Autodesk Inventor part; units mm, degrees
ref_plane "YZ Plane" through (0, 0, 0) normal (1, 0, 0) x (0, 1, 0)
ref_plane "XZ Plane" through (0, 0, 0) normal (0, 1, 0) x (-1, 0, 0)
ref_plane "XY Plane" through (0, 0, 0) normal (0, 0, 1) x (1, 0, 0)
sketch "Szkic1" plane through (0, 0, 0) normal (1, 0, 0) x (0, 1, 0)
  circle A0 centre (0, 0) radius 8
  dimension "d0" = 16
extrude "Wyciągnięcie proste1" add sketch "Szkic1" along normal mid plane 15
sketch "Szkic2" plane through (7.5, 0, 0) normal (1, 0, 0) x (0, 0, -1)
  circle A0 centre (-2, 0) radius 3.5
  point P0 (0, 0)
  dimension "d3" = 7
  dimension "d4" = 2
extrude "Wyciągnięcie proste2" add sketch "Szkic2" along normal blind 1
mirror "Odbij1" about plane through (0, 0, 0) normal (1, 0, 0) of "Wyciągnięcie proste2", "Wyciągnięcie proste1"
sketch "Szkic3" plane through (7.5, 0, 0) normal (1, 0, 0) x (0, 0, -1)
  point P0 (0, 0)
sketch "Szkic4" plane through (8.5, 0, 2) normal (1, 0, 0) x (0, 0, -1)
  circle A0 centre (2, 0) radius 8
  circle A1 centre (0, 0) radius 3.5
  point P0 (-6, 0)
  point P1 (-3.5, 0)
sketch "Szkic8" plane through (-7.5, 0, 0) normal (-1, 0, 0) x (0, 0, 1)
  circle A0 centre (0, 0) radius 8
  line L0 (8, 0) -> (5.5, 0)
  circle A1 centre (2, 0) radius 3.5
properties part number "Przekładnia rolka" material "Stal"
Geometry check sheet. Reference: the model listing, model coordinates, mm. A direction names the side the tool comes from. Coordinates: 2 decimals unless noted, no trailing zeros. Write each loop counter-clockwise with the first axis right and the second up, starting at its lowest first coordinate (ties: lowest second). Pieces come first, ordered by that corner, then holes. Notation, with made-up numbers: M 41.25,66 L 71.25,66 A20 cw 71.25,99 Z; hole C 17,38.25 d3. An arc over 180 degrees is marked long. Answer as a JSON object with one key per item and string values.
1. Scan lines: L1, parallel to X at y = -2.25, z = -2.5; L2, parallel to Y at x = 6, z = -3.5; L3, parallel to Z at x = -0.5, y = 7. Record each from-to range of solid material in increasing order.
Answers below:
{"L1": "x = -7.5 to 7.5", "L2": "y = -7.19 to 7.19", "L3": "z = -3.87 to 3.87"}
2. Tool access check on faces 1 (the cylindrical face through (0.11, -1.73, -7.81)), 2 (the cylindrical face through (7.993, 1.341, -1.233)), 3 (the flat face through (-7.5, 0, -2)). Record the directions out of +Z, -Z, +X, -X, +Y, -Y that give a thin tool (end or side, any length) a straight path to the whole face; none if there is none.
Answers below:
{"face 1": "+X, -X", "face 2": "+X", "face 3": "-X"}
3. Go/stop test with a flat-tipped pin: pin 1 Ø8 at (y, z) = (-3.5, -5.5) entering from -X. Record where the tip stops, or that it passes through.
Answers below:
{"pin 1": "stops at x = -7.5"}
4. Section check D-D, the plane z = 6. Enter the section's corners in (x, y).
Answers below:
{"outline": "M -7.5,-5.29 L 7.5,-5.29 L 7.5,5.29 L -7.5,5.29 Z"}
5. Section check A-A, the plane y = 0. Enter the section's corners in (x, z), plus the area to 3 significant figures.
Answers below:
{"outline": "M -8.5,-1.5 L -7.5,-1.5 L -7.5,-8 L 7.5,-8 L 7.5,-1.5 L 8.5,-1.5 L 8.5,5.5 L 7.5,5.5 L 7.5,8 L -7.5,8 L -7.5,5.5 L -8.5,5.5 Z", "area": "254 mm²"}
6. Section check C-C, the plane x = -1.75. Enter the section's corners in (y, z), plus the area to 3 significant figures.
Answers below:
{"outline": "C 0,0 d16", "area": "201 mm²"}
7. Section check B-B, the plane z = 3.75. Enter the section's corners in (x, y), plus the area to 3 significant figures.
Answers below:
{"outline": "M -8.5,-3.03 L -7.5,-3.03 L -7.5,-7.07 L 7.5,-7.07 L 7.5,-3.03 L 8.5,-3.03 L 8.5,3.03 L 7.5,3.03 L 7.5,7.07 L -7.5,7.07 L -7.5,3.03 L -8.5,3.03 Z", "area": "224 mm²"}
